Job drawing, mm, ordinate dimensions from the low corner. One solid piece. A direction names the side the tool comes from. Give positions to 0.01 mm unless a question says otherwise; leave off trailing zeros. Loops run counter-clockwise (first coordinate to the right, second up) from the corner with the lowest first, then second, coordinate; pieces in that order, holes last. Notation, with made-up numbers: M 53.25,70.5 L 74.25,70.5 A36 ccw 74.25,104.5 Z; hole C -8.75,55 d1. An arc over 180 degrees is marked long. Answer in a Markdown table with one row per item.
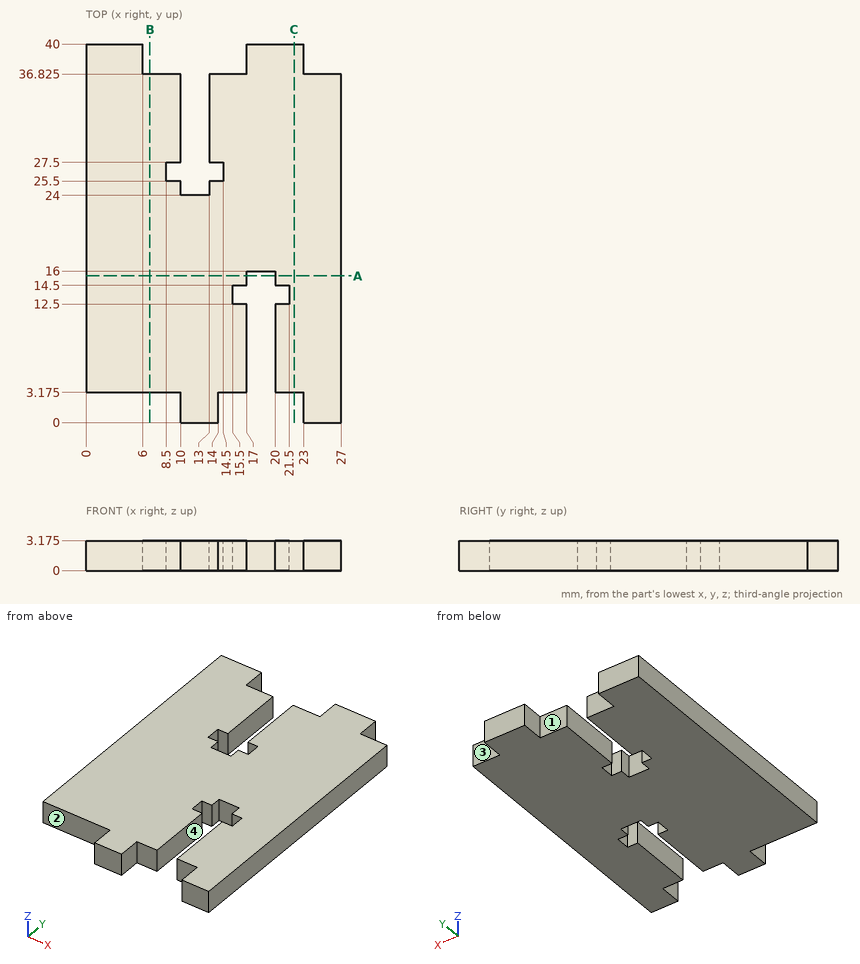
(1) Drill centre lines: line 1 along X through (y, z) = (28.5, 1.9); line 2 along X through (y, z) = (11, 1.25); line 3 along Y through (x, z) = (21, 1.3) (3 decimals). Where is each one in solid material? Low to high.
Recorded:
| item | result |
|---|---|
| line 1 | x = 0 to 10, 13 to 27 |
| line 2 | x = 0 to 17, 20 to 27 |
| line 3 | y = 3.175 to 12.5, 14.5 to 40 |
(2) Pin check, flat tips, straight feed: pin 1 Ø1.6 at (x, z) = (16, 1) entering from +Y (3 decimals); pin 2 Ø1.2 at (x, z) = (20.5, 2) entering from -Y (3 decimals); pin 3 Ø1.5 at (x, z) = (11.5, 1) entering from +Y. Stop position of each tip, or through.
Recorded:
| item | result |
|---|---|
| pin 1 | stops at y = 36.825 |
| pin 2 | stops at y = 3.175 |
| pin 3 | stops at y = 24 |
(3) Saw through at C-C (x = 22). Write the cut outline in (y, z) (3 decimals), plus the area to 3 significant figures.
Recorded:
| item | result |
|---|---|
| outline | M 3.175,0 L 40,0 L 40,3.175 L 3.175,3.175 Z |
| area | 117 mm^2 |
(4) Saw through at A-A (y = 15.5). Write the cut outline in (x, z) (3 decimals).
Recorded:
| item | result |
|---|---|
| outline | M 0,0 L 17,0 L 17,3.175 L 0,3.175 Z; M 20,0 L 27,0 L 27,3.175 L 20,3.175 Z |
(5) Which spindle directions (+Z, -Z, +X, -X, +Y, -Y) get a long thin tool onto all of the face, cutting with end or side? Do the marked faces 1, 2, 3 and 4. Say none if no direction does.
Recorded:
| item | result |
|---|---|
| face 1 | +Z, -Z, +Y |
| face 2 | +Z, -Z, -X, -Y |
| face 3 | +Z, -Z, +X, +Y |
| face 4 | +Z, -Z, -Y |
(6) Saw through at B-B (x = 6.75). Write the cut outline in (y, z) (3 decimals), plus the area to 3 significant figures.
Recorded:
| item | result |
|---|---|
| outline | M 3.175,0 L 36.825,0 L 36.825,3.175 L 3.175,3.175 Z |
| area | 107 mm^2 |
